```python
from build123d import *

# Parameters (mm, degrees)
F0_R     = 11
F0_R_2   = 5.5
F1_DEPTH = 1
F0_R_3   = 4.75
F0_R_4   = 4.5
F2_DEPTH = 1.4
F3_DEPTH = 5
F4_DEPTH = 1


with BuildPart() as f1:
    # F0 (on Top) → F1 (new body)
    with BuildSketch(Plane.XY):
        Circle(F0_R)
        Circle(F0_R_2, mode=Mode.SUBTRACT)
    extrude(amount=F1_DEPTH)

    # F0 (on Top) → F2 (join)
    with BuildSketch(Plane.XY):
        Circle(F0_R_2)
        Circle(F0_R_3, mode=Mode.SUBTRACT)
        Circle(F0_R_3)
        Circle(F0_R_4, mode=Mode.SUBTRACT)
    extrude(amount=F2_DEPTH)

    # F0 (on Top) → F3 (join)
    with BuildSketch(Plane.XY):
        Circle(F0_R_3)
        Circle(F0_R_4, mode=Mode.SUBTRACT)
    extrude(amount=F3_DEPTH)

    # F0 (on Top) → F4 (join)
    with BuildSketch(Plane.XY):
        Circle(F0_R_4)
    extrude(amount=F4_DEPTH)


solid = f1.part
```
Here's how the part is built. I have some questions about the finished solid (model axes, mm). A direction names the side the tool comes from. Coordinates: 2 decimals unless noted, no trailing zeros. Write each loop counter-clockwise with the first axis right and the second up, starting at its lowest first coordinate (ties: lowest second). Pieces come first, ordered by that corner, then holes. Notation, with made-up numbers: M 83,-8 L 128,-8 A20 ccw 128,28 Z; hole C 67,56.5 d4. An arc over 180 degrees is marked long. Answer as CSV lines item,"result". Start each with the question number.
Q1. Suppose I cut it at A-A, the plane x = 0. List the corners of the cut face in (y, z) for me.
Q2. For faces 1 (the flat face through (0, 0, 1)), 2 (the cylindrical face through (-2.38, -10.74, 0.49)), which set-ups out of +Z, -Z, +X, -X, +Y, -Y let a thin tool reach every point of the face, with its end or its side?
Q3. Suppose I cut it at C-C, the plane z = 2.8. List the corners of the cut face in (x, y) for me, then the cut area to 3 significant figures.
Q4. If we mould it in two halves opening along X, with no side actions, what happens to faces 3 (the cylindrical face through (-0.59, 4.46, 2.97)), 4 (the cylindrical face through (2.192, -4.214, 3.175)), 5 (the flat face through (0, 0, 0))? For each: pulls with the +X half, pulls with the -X half, needs draft (parallel to the pull), parting line crosses it, or undercut.
Q5. Suppose I cut it at D-D, the plane z = 0.6. List the corners of the cut face in (x, y) for me.
Q6. I need wall thicknesses on probe 1 along Y at (x, z) = (0, 3.15); probe 2 along Z at (x, y) = (-7, 4); probe 3 along Y at (x, z) = (-1, 3.6). Which ranges of each line are inside material? Lowest first, please. Write a range as [from, to].
Q7. Will these pins go through, and if not, where does the flat tip stop? pin 1 Ø1.5 at (y, z) = (3, 0.5) entering from -X; pin 2 Ø1 at (x, y) = (-8, 6) entering from +Z.
Entries:
1,outline,"M -11,0 L 11,0 L 11,1 L 5.5,1 L 5.5,1.4 L 4.75,1.4 L 4.75,5 L 4.5,5 L 4.5,1 L -4.5,1 L -4.5,5 L -4.75,5 L -4.75,1.4 L -5.5,1.4 L -5.5,1 L -11,1 Z"
2,face 1,"+Z"
2,face 2,"+Z, -Z"
3,outline,"C 0,0 d9.5; hole C 0,0 d9"
3,area,"7.26 mm²"
4,face 3,"undercut"
4,face 4,"parting line crosses it"
4,face 5,"needs draft"
5,outline,"C 0,0 d22"
6,probe 1,"y = [-4.75, -4.5], [4.5, 4.75]"
6,probe 2,"z = [0, 1]"
6,probe 3,"y = [-4.64, -4.39], [4.39, 4.64]"
7,pin 1,"stops at x = -10.77"
7,pin 2,"stops at z = 1"
